Build history of the part. All positions in model axes, mm. Face numbers are marked on the shaded views. A direction names the side the tool comes from. Coordinates: 2 decimals unless noted, no trailing zeros. Loops run counter-clockwise (first coordinate to the right, second up) from the corner with the lowest first, then second, coordinate; pieces in that order, holes last. Notation, with made-up numbers: (83, -17.5) -> (128, -17.5) arc R25 cw to (128, 3.5) -> close; hole circle Ø7 at (52.25, 35.5). An arc over 180 degrees is marked (long way). One line per item, written item: value. Start each with the question number.
```python
from build123d import *

# Parameters (mm, degrees)
SKETCH1_R           = 10
BOSS_EXTRUDE1_DEPTH = 20
BOSS_EXTRUDE2_START = 4
BOSS_EXTRUDE2_DEPTH = 4


with BuildPart() as part:
    # Sketch1 → Boss-Extrude1 (new body)
    with BuildSketch(Plane(origin=(0, 0, 0), x_dir=(1, 0, 0), z_dir=(0, 1, 0))):
        with BuildLine():
            Line((5.103736684, -12.52406407), (20, -12.52406407))
            Line((20, -12.52406407), (20, -14.52406407))
            Line((20, -14.52406407), (-20, -14.52406407))
            Line((-20, -14.52406407), (-20, -12.52406407))
            Line((-20, -12.52406407), (-5.103736684, -12.52406407))
            ThreePointArc((-5.103736684, -12.52406407), (0, 13.52406407), (5.103736684, -12.52406407))
        make_face()
        with Locations(Location((0, 0, 0), (0, 0, 270))):
            Circle(SKETCH1_R, mode=Mode.SUBTRACT)
    extrude(amount=BOSS_EXTRUDE1_DEPTH)

    # Sketch2 → Boss-Extrude2 (add)
    with BuildSketch(Plane.XZ.offset(BOSS_EXTRUDE2_START)):
        with BuildLine():
            Line((5.103736684, 12.52406407), (20, 12.52406407))
            Line((20, 12.52406407), (20, 14.52406407))
            Line((20, 14.52406407), (-20, 14.52406407))
            Line((-20, 14.52406407), (-20, 12.52406407))
            Line((-20, 12.52406407), (-5.103736684, 12.52406407))
            ThreePointArc((-5.103736684, 12.52406407), (0, -13.52406407), (5.103736684, 12.52406407))
        make_face()
    extrude(amount=-BOSS_EXTRUDE2_DEPTH)


solid = part.part
```
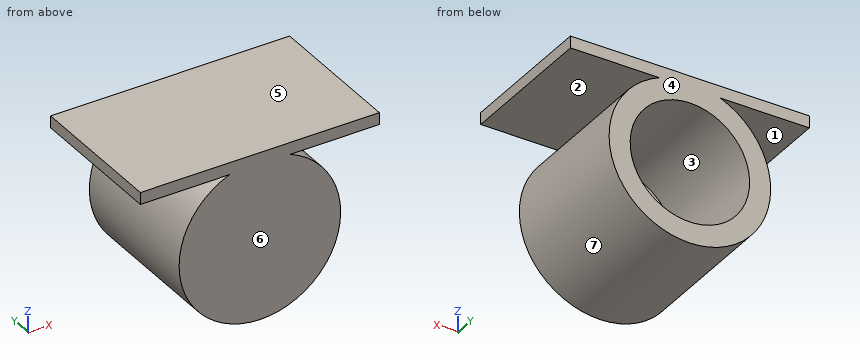
Item 1: Probe probe 1 along X at (y, z) = (9.75, 0); probe 2 along Z at (x, y) = (6, 7.75); probe 3 along Z at (x, y) = (-14, 16.5). List the from-to ranges inside material, lowest first.
Item 2: Drop flat-ended pins along their axis: pin 1 Ø6 at (y, z) = (11.5, 1) entering from +X; pin 2 Ø6 at (x, z) = (0.5, -3) entering from +Y; pin 3 Ø12 at (x, y) = (-13, 7.5) entering from -Z. Give the stop position or say it passes through.
Item 3: Band-saw the part on D-D, the plane x = 0. List the corners of the cut face in (y, z), and give its area (3 significant figures).
Item 4: Tool access for the marked faces 1, 2, 3 and 4: list every direction of +Z, -Z, +X, -X, +Y, -Y with a clear straight run to the whole face (end or side of a thin tool).
Item 5: Band-saw the part on B-B, the plane x = -13. List the corners of the cut face in (y, z), and give its area (3 significant figures).
Item 6: Band-saw the part on C-C, the plane z = 0. List the corners of the cut face in (x, y).
Item 7: Two-plate mould, pull along Z, no slides. Class the marked faces 5, 6 and 7: +Z half, -Z half, draft (parallel to the pull), parting line (faces both ways), or undercut.
Item 8: Band-saw the part on A-A, the plane y = 6.75. List the corners of the cut face in (x, z), and give its area (3 significant figures).
Worked out:
1. probe 1: x = -13.52 to -10, 10 to 13.52
1. probe 2: z = -12.12 to -8, 8 to 12.12, 12.52 to 14.52
1. probe 3: z = 12.52 to 14.52
2. pin 1: stops at x = 13.52
2. pin 2: stops at y = 0
2. pin 3: stops at z = -11.57
3. outline: (-4, -13.52) -> (20, -13.52) -> (20, -10) -> (0, -10) -> (0, 10) -> (20, 10) -> (20, 14.52) -> (-4, 14.52) -> close
3. area: 273 mm²
4. face 1: -X, +Y, -Y
4. face 2: +X, +Y, -Y
4. face 3: +Y
4. face 4: +Z, -Z, +X, -X, +Y
5. outline: (-4, -3.73) -> (20, -3.73) -> (20, 3.73) -> (-4, 3.73) -> close; (-4, 12.52) -> (20, 12.52) -> (20, 14.52) -> (-4, 14.52) -> close
5. area: 227 mm²
6. outline: (-13.52, -4) -> (13.52, -4) -> (13.52, 20) -> (10, 20) -> (10, 0) -> (-10, 0) -> (-10, 20) -> (-13.52, 20) -> close
7. face 5: +Z half
7. face 6: draft
7. face 7: undercut
8. outline: (-20, 12.52) -> (-5.1, 12.52) arc R13.52 ccw (long way) to (5.1, 12.52) -> (20, 12.52) -> (20, 14.52) -> (-20, 14.52) -> close; hole circle Ø20 at (0, 0)
8. area: 334 mm²
